Can you work these out from the model? Positions are in its coordinate system, mm. Face numbers are marked on the shaded views. A direction names the side the tool comes from. Coordinates: 2 decimals unless noted, no trailing zeros. Order: outer loops, then holes, each group sorted by start corner. A loop starts at its lowest first (then second) coordinate and runs counter-clockwise, first axis right, second up. Notation, with made-up numbers: (-22.5, -33.75) -> (18.5, -33.75) arc R24 cw to (18.5, -10.75) -> close; hole circle Ø3 at (71.5, 24). An arc over 180 degrees is marked (long way). Answer in a Markdown table with one row per item.
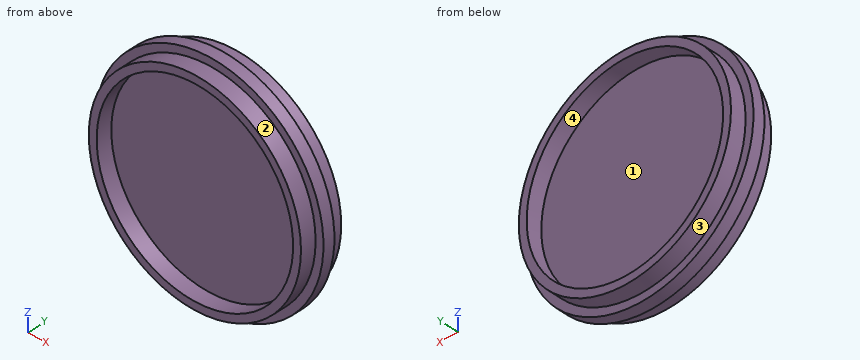
```python
from build123d import *

# Parameters (mm, degrees)
SKETCH1_W           = 127.635
SKETCH1_H           = 127.635
BOSS_EXTRUDE1_DEPTH = 9.525
SKETCH12_R          = 92.075
BOSS_EXTRUDE2_DEPTH = 9.525
SKETCH30_R          = 85.725
SKETCH30_R_2        = 79.375
BOSS_EXTRUDE3_DEPTH = 12.7


with BuildPart() as part:
    # Sketch1 → Boss-Extrude1 (new body)
    with BuildSketch(Plane(origin=(0, 0, 0), x_dir=(1, 0, 0), z_dir=(0, 1, 0))):
        with Locations((63.8175, 63.8175)):
            Rectangle(SKETCH1_W, SKETCH1_H)
    extrude(amount=BOSS_EXTRUDE1_DEPTH)

    # Sketch12 → Boss-Extrude2 (add)
    with BuildSketch(Plane.XZ):
        with Locations(Location((63.8175, -63.8175, 0), (0, 0, 270))):
            Circle(SKETCH12_R)
    extrude(amount=-BOSS_EXTRUDE2_DEPTH)

    # Sketch30 → Boss-Extrude3 (add)
    with BuildSketch(Plane.XZ):
        with Locations(Location((63.8175, -63.8175, 0), (0, 0, 270))):
            Circle(SKETCH30_R)
        with Locations(Location((63.8175, -63.8175, 0), (0, 0, 270))):
            Circle(SKETCH30_R_2, mode=Mode.SUBTRACT)
    boss_extrude3 = extrude(amount=BOSS_EXTRUDE3_DEPTH)

    # Mirror1: Boss-Extrude3 across plane
    add(boss_extrude3.mirror(Plane.ZX.offset(4.7625)))


solid = part.part
```
(1) Will these pins go through, and if not, where does the flat tip stop? pin 1 Ø1 at (x, z) = (78, 9) entering from +Y (3 decimals); pin 2 Ø2 at (x, y) = (45, 2) entering from +Z; pin 3 Ø5 at (y, z) = (-3, -3.5) entering from -X.
Response values:
| item | result |
|---|---|
| pin 1 | y = 9.525 |
| pin 2 | z = 26.52 |
| pin 3 | x = 0.53 |
(2) I need wall thicknesses on line 1 (Z direction, x = 112.5, y = -7); line 2 (Y direction, x = 75.5, z = -96) (3 decimals); line 3 (X direction, y = -8, z = -12). Which ranges of each line are inside material? Lowest first, please. Write a range as [from, to].
Response values:
| item | result |
|---|---|
| line 1 | [-134.38, -126.51], [-1.12, 6.74] |
| line 2 | [0, 9.525] |
| line 3 | [-4.47, 3.69], [123.95, 132.11] |
(3) Suppose I cut it at B-B (z = -23.5). Please give me the cut outline in (x, y) (3 decimals).
Response values:
| item | result |
|---|---|
| outline | (-18.961, 0) -> (-11.835, 0) -> (-11.835, -12.7) -> (-4.556, -12.7) -> (-4.556, 0) -> (132.191, 0) -> (132.191, -12.7) -> (139.47, -12.7) -> (139.47, 0) -> (146.596, 0) -> (146.596, 9.525) -> (139.47, 9.525) -> (139.47, 22.225) -> (132.191, 22.225) -> (132.191, 9.525) -> (-4.556, 9.525) -> (-4.556, 22.225) -> (-11.835, 22.225) -> (-11.835, 9.525) -> (-18.961, 9.525) -> close |
(4) We'd pull the mould along X, two halves only. Please class the marked faces 3 and 4: +X half, -X half, draft (parallel to the pull), parting line (faces both ways), or undercut.
Response values:
| item | result |
|---|---|
| face 3 | parting line |
| face 4 | undercut |
(5) On a 3-axis mill with a long thin cutter (end or side, diameter ignored), from which of +Z, -Z, +X, -X, +Y, -Y can I reach the whole of each face in a straight line? I mean the marked faces 1 and 2. Say none if no direction works.
Response values:
| item | result |
|---|---|
| face 1 | +Y |
| face 2 | -Y |
(6) Suppose I cut it at A-A (x = 93.5). Please give me the cut outline in (y, z) (3 decimals), and give its area (3 significant figures).
Response values:
| item | result |
|---|---|
| outline | (-12.7, -144.24) -> (0, -144.24) -> (0, -150.977) -> (9.525, -150.977) -> (9.525, -144.24) -> (22.225, -144.24) -> (22.225, -137.434) -> (9.525, -137.434) -> (9.525, 9.799) -> (22.225, 9.799) -> (22.225, 16.605) -> (9.525, 16.605) -> (9.525, 23.342) -> (0, 23.342) -> (0, 16.605) -> (-12.7, 16.605) -> (-12.7, 9.799) -> (0, 9.799) -> (0, -137.434) -> (-12.7, -137.434) -> close |
| area | 2,010 mm2 |
